Could you check a few things on this model? Use its own coordinates, in mm. A direction names the side the tool comes from. Give positions to 0.01 mm unless a question says otherwise; leave off trailing zeros. Order: outer loops, then holes, each group sorted by start corner. A loop starts at its lowest first (then second) coordinate and runs counter-clockwise, first axis right, second up. Notation, with made-up numbers: (-29, 82) -> (8, 82) arc R24 ccw to (8, 120) -> close; hole circle Ø1 at (4, -27). An arc over 180 degrees is marked (long way). One line per item, written item: value.
```python
from build123d import *

# Parameters (mm, degrees)
SKETCH1_R           = 1.65
BOSS_EXTRUDE1_DEPTH = 4
SKETCH2_W           = 2.2
SKETCH2_H           = 8
BOSS_EXTRUDE2_DEPTH = 4
FILLET1_R           = 1
FILLET2_R           = 1
BOSS_EXTRUDE3_DEPTH = 4


with BuildPart() as part:
    # Sketch1 → Boss-Extrude1 (new body)
    with BuildSketch(Plane(origin=(0, 0, 0), x_dir=(1, 0, 0), z_dir=(0, 1, 0))):
        Polygon((4.781972019, 3), (-7.218027981, 0), (-7.218027981, -5), (-1.218027981, -5), (4.781972019, -1.5), (4.781972019, 0), align=None)
        with Locations(Location((-4.78871413, -1.763457272, 0), (0, 0, 270))):
            Circle(SKETCH1_R, mode=Mode.SUBTRACT)
    extrude(amount=BOSS_EXTRUDE1_DEPTH)

    # Sketch2 → Boss-Extrude2 (add)
    with BuildSketch(Plane(origin=(0, 4, 0), x_dir=(1, 0, 0), z_dir=(0, 1, 0))):
        with Locations((-2.318027981, -9)):
            Rectangle(SKETCH2_W, SKETCH2_H)
    extrude(amount=-BOSS_EXTRUDE2_DEPTH)

    # Fillet1
    fillet1_edges = [part.edges().sort_by_distance(p)[0] for p in [
        (-1.218027981, 2, 13),
        (-3.418027981, 2, 13),
    ]]
    fillet(fillet1_edges, radius=FILLET1_R)

    # Fillet2
    fillet2_edges = [part.edges().sort_by_distance(p)[0] for p in [
        (-7.218027981, 2, 5),
    ]]
    fillet(fillet2_edges, radius=FILLET2_R)

    # Sketch3 → Boss-Extrude3 (add)
    with BuildSketch(Plane(origin=(0, 4, 0), x_dir=(1, 0, 0), z_dir=(0, 1, 0))):
        Polygon((-7.218027981, 0), (-8.479213231, -0.315296313), (-7.218027981, -4), align=None)
    extrude(amount=-BOSS_EXTRUDE3_DEPTH)


solid = part.part
```
1) For faces 4 (the flat face through (-1.218, 2, 9)), 5 (the flat face through (-2, 4, 3)), 6 (the flat face through (-3.418, 2, 9)), which set-ups out of +Z, -Z, +X, -X, +Y, -Y let a thin tool reach every point of the face, with its end or its side?
Answer below:
face 4: +Z, +X, +Y, -Y
face 5: +Z, -Z, +X, -X, +Y
face 6: +Z, -X, +Y, -Y
2) Suppose I cut it at D-D, the plane z = 7. Write out the boundary of the cut face in (x, y).
Answer below:
outline: (-3.42, 0) -> (-1.22, 0) -> (-1.22, 4) -> (-3.42, 4) -> close
3) We'd pull the mould along Z, two halves only. Please class faces 1 (the flat face through (4.782, 2, -1)), 2 (the cylindrical face through (-3.397, 1.972, 2.65)), 3 (the flat face through (-7.86, 2.03, 2.13)): +Z half, -Z half, draft (parallel to the pull), parting line (faces both ways), or undercut.
Answer below:
face 1: draft
face 2: undercut
face 3: +Z half
4) Suppose I cut it at A-A, the plane z = 2. Write out the boundary of the cut face in (x, y).
Answer below:
outline: (-7.9, 0) -> (-6.42, 0) -> (-6.42, 4) -> (-7.9, 4) -> close; (-3.16, 0) -> (3.92, 0) -> (3.92, 4) -> (-3.16, 4) -> close
5) If I drill on line 1 along X through (y, z) = (1.8, 10); line 2 along Z through (x, y) = (-6, 3.05); line 3 along Z through (x, y) = (-6.25, 3.25), over which ranges is the centre line in solid material (lowest first)?
Answer below:
line 1: x = -3.42 to -1.22
line 2: z = -0.3 to 0.64, 2.88 to 5
line 3: z = -0.24 to 1, 2.53 to 5
6) For P1, Ø1.2, axis at y = 2.5, z = 10, coming from the -X side; P2, Ø2, axis at x = -5, z = 8.5, coming from the -Y side; P3, Ø2, axis at y = 1, z = 8, coming from the +X side; P4, Ø2, axis at x = -0.5, y = 1, coming from the -Z side, each with a flat end and sliding along its axis, tell me the tip position at first contact or that it passes through.
Answer below:
P1: stops at x = -3.42
P2: passes through
P3: stops at x = -1.22
P4: stops at z = -1.93
7) Suppose I cut it at C-C, the plane y = 2. Write out the boundary of the cut face in (x, z).
Answer below:
outline: (-8.48, 0.32) -> (4.78, -3) -> (4.78, 1.5) -> (-1.22, 5) -> (-1.22, 12) arc R1 ccw to (-2.22, 13) -> (-2.42, 13) arc R1 ccw to (-3.42, 12) -> (-3.42, 5) -> (-6.22, 5) arc R1 ccw to (-7.22, 4) -> close; hole circle Ø3.3 at (-4.79, 1.76)
8) Suppose I cut it at B-B, the plane x = -4.5. Write out the boundary of the cut face in (y, z).
Answer below:
outline: (0, -0.68) -> (4, -0.68) -> (4, 0.14) -> (0, 0.14) -> close; (0, 3.39) -> (4, 3.39) -> (4, 5) -> (0, 5) -> close
